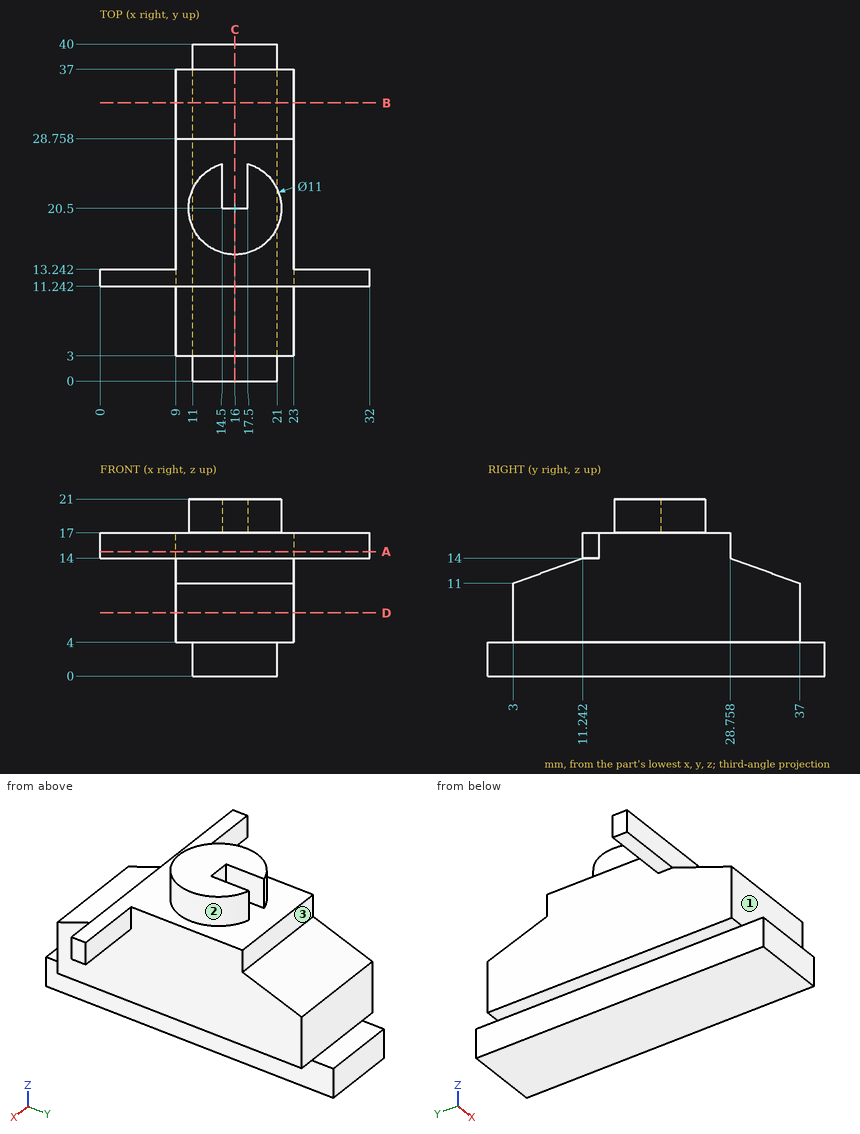
Study the drawing (mm; zero at the part's minimum x, y, z) and answer. A direction names the side the tool comes from. Round coordinates to 2 decimals unless told otherwise and drop trailing zeros. Write each loop counter-clockwise with the first axis right and the second up, starting at its lowest first coordinate (ties: lowest second). Pieces come first, ordered by that corner, then holes. Notation, with made-up numbers: (74.25, 77) -> (120.25, 77) arc R13 ccw to (120.25, 90) -> close; hole circle Ø8 at (28, -35.5). An arc over 180 degrees is marked (long way). Write item = value, one per line.
1) Straight lines are drawn through the part: line 1 along Z through (x, y) = (16, 38); line 2 along Y through (x, z) = (20, 8.5); line 3 along X through (y, z) = (29, 13). For each, find the intervals that lie inside material, in ascending order. Write a range as [from, to].
Check values:
line_1 = [0, 4]
line_2 = [3, 37]
line_3 = [9, 23]
2) Section C-C on x = 16 is taken. Write down the section's boundary in (y, z), plus the area to 3 significant figures.
Check values:
outline = (0, 0) -> (40, 0) -> (40, 4) -> (37, 4) -> (37, 11) -> (28.76, 14) -> (28.76, 17) -> (20.5, 17) -> (20.5, 21) -> (15, 21) -> (15, 17) -> (11.24, 17) -> (11.24, 14) -> (3, 11) -> (3, 4) -> (0, 4) -> close
area = 550 mm²
3) Given pin 1 (6 mm diameter, centred on x = 23, z = 11.5, fed in from +Y); pin 2 (2.5 mm diameter, centred on x = 29.5, z = 16, fed in from +Y); pin 3 (3.5 mm diameter, centred on x = 12.5, z = 16, fed in from -Y), each flat-ended and moving along its own axis, determine where each tip first touches the part or whether it passes through.
Check values:
pin_1 = 37
pin_2 = 13.24
pin_3 = 11.24
4) Which of the six approach directions +Z, -Z, +X, -X, +Y, -Y give full straight-line access (tool end or side, diameter ignored) to the marked faces 1, 2 and 3?
Check values:
face_1 = +Z, +X, -X, -Y
face_2 = +Z
face_3 = +Z, +X, -X, +Y
5) Section D-D on z = 7.5 is taken. Write down the section's boundary in (x, y).
Check values:
outline = (9, 3) -> (23, 3) -> (23, 37) -> (9, 37) -> close
6) Section A-A on z = 14.75 is taken. Write down the section's boundary in (x, y), plus the area to 3 significant figures.
Check values:
outline = (0, 11.24) -> (32, 11.24) -> (32, 13.24) -> (23, 13.24) -> (23, 28.76) -> (9, 28.76) -> (9, 13.24) -> (0, 13.24) -> close
area = 281 mm²
7) Section B-B on y = 33 is taken. Write down the section's boundary in (x, z), plus the area to 3 significant figures.
Check values:
outline = (9, 4) -> (11, 4) -> (11, 0) -> (21, 0) -> (21, 4) -> (23, 4) -> (23, 12.46) -> (9, 12.46) -> close
area = 158 mm²
